Could you check a few things on this model? Use its own coordinates, in mm. A direction names the side the tool comes from. Coordinates: 2 decimals unless noted, no trailing zeros. Order: outer loops, then holes, each group sorted by start corner. A loop starts at its lowest first (then second) coordinate and runs counter-clockwise, first axis right, second up. Notation, with made-up numbers: M -13.75,89.25 L 20.25,89.25 A33 ccw 20.25,119.25 Z; hole C 5,27 d7. An arc over 180 degrees is marked long. Put each result on its own line as item: value. Start each with the question number.
```python
from build123d import *

# Parameters (mm, degrees)
SKETCH1_R           = 5.626
SKETCH1_R_2         = 4.826
BOSS_EXTRUDE1_DEPTH = 7.5
SKETCH2_R           = 10
SKETCH2_R_2         = 5.626
BOSS_EXTRUDE2_DEPTH = 1.5


with BuildPart() as part:
    # Sketch1 → Boss-Extrude1 (new body, symmetric)
    with BuildSketch(Plane(origin=(0, 0, 0), x_dir=(1, 0, 0), z_dir=(0, 1, 0))):
        Circle(SKETCH1_R)
        Circle(SKETCH1_R_2, mode=Mode.SUBTRACT)
    extrude(amount=BOSS_EXTRUDE1_DEPTH, both=True)

    # Sketch2 → Boss-Extrude2 (add)
    with BuildSketch(Plane(origin=(0, 7.5, 0), x_dir=(1, 0, 0), z_dir=(0, 1, 0))):
        Circle(SKETCH2_R)
        Circle(SKETCH2_R_2, mode=Mode.SUBTRACT)
    boss_extrude2 = extrude(amount=-BOSS_EXTRUDE2_DEPTH)

    # Mirror1: Boss-Extrude2 across plane
    add(boss_extrude2.mirror(Plane.ZX))


solid = part.part
```
Item 1: If we mould it in two halves opening along Y, with no side actions, what happens to faces 1 (the cylindrical face through (-2.17, 6.76, 9.76)), 2 (the flat face through (2, 7.5, -5)), 3 (the flat face through (4.3, -6, 4.3))? For each: released by +Y, released by -Y, zero draft, split by the parting line, or undercut.
Item 2: For faces 4 (the cylindrical face through (-3.83, -0.105, 2.937)), 5 (the flat face through (4.3, 6, 4.3)), which set-ups out of +Z, -Z, +X, -X, +Y, -Y let a thin tool reach every point of the face, with its end or its side?
Item 3: For pin 1 Ø3 at (x, y) = (3.5, 2.5) entering from -Z; pin 2 Ø8.5 at (x, z) = (0, 0) entering from +Y; pin 3 Ø6 at (x, y) = (5.5, -2) entering from +Z; pin 4 Ø8 at (x, y) = (-8, 3) entering from -Z, each with a flat end and sliding along its axis, tell me the tip position at first contact or that it passes through.
Item 4: If we section it at A-A on x = 0: Write out the boundary of the cut face in (y, z), then the cut area to 3 significant figures.
Item 5: If we section it at B-B on z = 0: Write out the boundary of the cut face in (x, y).
Item 6: If we section it at C-C on x = 6: Write out the boundary of the cut face in (y, z), then the cut area to 3 significant figures.
Item 7: I need wall thicknesses on probe 1 along Z at (x, y) = (0, 1.25); probe 2 along Y at (x, z) = (-5, 6). Which ranges of each line are inside material? Lowest first, please.
Item 8: If we section it at D-D on y = 3.75: Write out the boundary of the cut face in (x, z).
Geometry check:
1. face 1: zero draft
1. face 2: released by +Y
1. face 3: undercut
2. face 4: +Y, -Y
2. face 5: none
3. pin 1: stops at z = -5.26
3. pin 2: passes through
3. pin 3: stops at z = 5.04
3. pin 4: stops at z = -8.45
4. outline: M -7.5,-10 L -6,-10 L -6,-5.63 L 6,-5.63 L 6,-10 L 7.5,-10 L 7.5,-4.83 L -7.5,-4.83 Z; M -7.5,4.83 L 7.5,4.83 L 7.5,10 L 6,10 L 6,5.63 L -6,5.63 L -6,10 L -7.5,10 Z
4. area: 50.2 mm²
5. outline: M -10,-7.5 L -4.83,-7.5 L -4.83,7.5 L -10,7.5 L -10,6 L -5.63,6 L -5.63,-6 L -10,-6 Z; M 4.83,-7.5 L 10,-7.5 L 10,-6 L 5.63,-6 L 5.63,6 L 10,6 L 10,7.5 L 4.83,7.5 Z
6. outline: M -7.5,-8 L -6,-8 L -6,8 L -7.5,8 Z; M 6,-8 L 7.5,-8 L 7.5,8 L 6,8 Z
6. area: 48.0 mm²
7. probe 1: z = -5.63 to -4.83, 4.83 to 5.63
7. probe 2: y = -7.5 to -6, 6 to 7.5
8. outline: C 0,0 d11.25; hole C 0,0 d9.65
